Source: CAD feature listing. Evaluate the final solid. Frame: model axes, mm. Face numbers are marked on the shaded views. A direction names the side the tool comes from. Give positions to 0.01 mm unless a question says otherwise; leave off trailing zeros. Loops run counter-clockwise (first coordinate to the right, second up) from the corner with the lowest first, then second, coordinate; pieces in that order, holes last. Notation, with made-up numbers: (-15, 33) - (36, 33) arc R33 cw to (36, 61) - close; hole circle Ø10 at (79.5, 79.5). An arc over 180 degrees is marked (long way). Put each result on its own line as item: value.
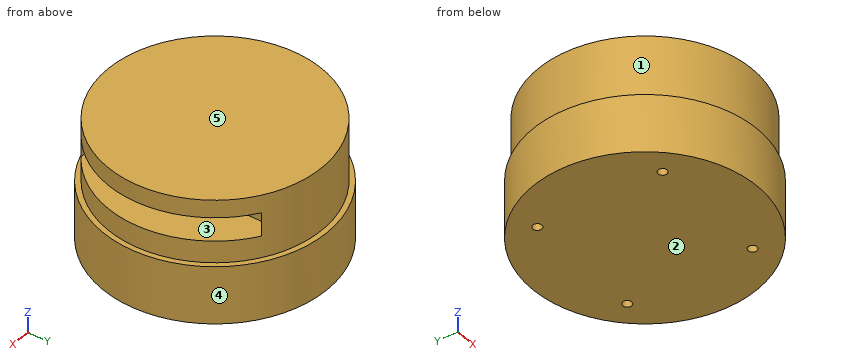
```python
from build123d import *

# Parameters (mm, degrees)
SKETCH_1_R          = 38
EXTRUDE_1_DEPTH     = 19.6
SKETCH_2_R          = 36.25
EXTRUDE_2_DEPTH     = 21.4
SKETCH_3_R          = 1.5
CUT_EXTRUDE_1_DEPTH = 4
CUT_EXTRUDE_2_REACH = 55
CUT_EXTRUDE_START   = 15
SKETCH_5_W          = 8
SKETCH_5_H          = 60


with BuildPart() as part:
    # 草图1 → 凸台-拉伸1 (new body)
    with BuildSketch(Plane.XY):
        Circle(SKETCH_1_R)
    extrude(amount=EXTRUDE_1_DEPTH)

    # 草图2 → 凸台-拉伸2 (add)
    with BuildSketch(Plane.XY.offset(19.6)):
        Circle(SKETCH_2_R)
    extrude(amount=EXTRUDE_2_DEPTH)

    # 草图3 → 切除-拉伸1 (cut)
    with BuildSketch(Plane(origin=(0, 0, 0), x_dir=(-1, 0, 0), z_dir=(0, 0, -1))):
        with Locations((20.859650045, 20.859650045)):
            Circle(SKETCH_3_R)
        with Locations((20.859650045, -20.859650045)):
            Circle(SKETCH_3_R)
        with Locations((-20.859650045, -20.859650045)):
            Circle(SKETCH_3_R)
        with Locations((-20.859650045, 20.859650045)):
            Circle(SKETCH_3_R)
    extrude(amount=-CUT_EXTRUDE_1_DEPTH, mode=Mode.SUBTRACT)

    # 草图5 → 切除-拉伸2 (cut, up to next)
    with BuildSketch(Plane(origin=(0, 0, 0), x_dir=(0, 0, -1), z_dir=(1, 0, 0)).offset(CUT_EXTRUDE_START), mode=Mode.PRIVATE) as cut_extrude_2_sk1:
        with Locations((-31, 0)):
            Rectangle(SKETCH_5_W, SKETCH_5_H)
    cut_extrude_2_tool1 = extrude(cut_extrude_2_sk1.sketch, amount=CUT_EXTRUDE_2_REACH, mode=Mode.PRIVATE) & part.part
    add(cut_extrude_2_tool1.solids().sort_by_distance((15, 0, 31))[0], mode=Mode.SUBTRACT)


solid = part.part
```
1) Section query D-D, the plane x = 25. Output: boundary loops of the cut face in (y, z), plus the area to 3 significant figures.
Check result:
outline: (-28.62, 0) - (28.62, 0) - (28.62, 19.6) - (26.25, 19.6) - (26.25, 27) - (-26.25, 27) - (-26.25, 19.6) - (-28.62, 19.6) - close; (-26.25, 35) - (26.25, 35) - (26.25, 41) - (-26.25, 41) - close
area: 1,830 mm²
2) Section query A-A, the plane x = 0. Output: boundary loops of the cut face in (y, z).
Check result:
outline: (-38, 0) - (38, 0) - (38, 19.6) - (36.25, 19.6) - (36.25, 41) - (-36.25, 41) - (-36.25, 19.6) - (-38, 19.6) - close
3) Section query B-B, the plane y = 0. Output: boundary loops of the cut face in (x, z), plus the area to 3 significant figures.
Check result:
outline: (-38, 0) - (38, 0) - (38, 19.6) - (36.25, 19.6) - (36.25, 27) - (15, 27) - (15, 35) - (36.25, 35) - (36.25, 41) - (-36.25, 41) - (-36.25, 19.6) - (-38, 19.6) - close
area: 2,870 mm²
4) Mould query, pull axis Y, two halves, no side actions, for the marked faces 3, 4 and 5. Classes: pulls with the +Y half, pulls with the -Y half, needs draft (parallel to the pull), parting line crosses it, or undercut.
Check result:
face 3: undercut
face 4: parting line crosses it
face 5: needs draft
5) Material intervals for line 1 along Z through (x, y) = (21, -16.5); line 2 along Z through (x, y) = (-14, 33.5); line 3 along Y through (x, z) = (-1, 20.5), sorted ascending. Write a range as [from, to].
Check result:
line 1: [0, 27], [35, 41]
line 2: [0, 19.6]
line 3: [-36.24, 36.24]
6) Section query C-C, the plane x = 16. Output: boundary loops of the cut face in (y, z), plus the area to 3 significant figures.
Check result:
outline: (-34.47, 0) - (34.47, 0) - (34.47, 19.6) - (32.53, 19.6) - (32.53, 41) - (-32.53, 41) - (-32.53, 19.6) - (-34.47, 19.6) - close; hole (-30, 27) - (30, 27) - (30, 35) - (-30, 35) - close
area: 2,260 mm²
7) Access query for the marked faces 1 and 2. Directions: +Z, -Z, +X, -X, +Y, -Y. A direction counts if a zero-diameter tool reaches every point of the face in a straight line with its end or side. Return the directions, or none.
Check result:
face 1: +Z
face 2: -Z, +X, -X, +Y, -Y
8) Pin query (flat end, axial travel): P1, Ø8, axis at x = 24.5, z = 19.5, coming from the +Y side; P2, Ø1.5, axis at x = 20.5, y = -20.5, coming from the -Z side; P3, Ø3, axis at x = -0.5, z = 36, coming from the +Y side. Return the tip coordinate at first contact, or that it passes through.
Check result:
P1: y = 32
P2: z = 4
P3: y = 36.25
